from build123d import *

# Parameters (mm, degrees)
F0_R     = 10
F1_DEPTH = 20
F2_R     = 9
F3_DEPTH = 25


with BuildPart() as f1:
    # F0 (on Top) → F1 (new body)
    with BuildSketch(Plane.XY):
        with BuildLine():
            Line((0, -48.967767), (0, 0))
            Line((0, 0), (-150, 0))
            Line((-150, 0), (-150, -19.634434))
            ThreePointArc((-150, -19.634434), (-145.859777, -31.819157), (-135.153253, -38.959133))
            Line((-135.153253, -38.959133), (-25.153253, -68.292466))
            ThreePointArc((-25.153253, -68.292466), (-7.815277, -64.827544), (0, -48.967767))
        make_face()
        with Locations((-20, -48.967767)):
            Circle(F0_R, mode=Mode.SUBTRACT)
        with Locations((-130, -19.634434)):
            Circle(F0_R, mode=Mode.SUBTRACT)
    extrude(amount=F1_DEPTH)

    # F2 (on Front) → F3 (join)
    with BuildSketch(Plane.XZ):
        with BuildLine():
            Line((-84.449692, 0), (0, 0))
            Line((0, 0), (0, 35.662658))
            ThreePointArc((0, 35.662658), (-7.296527, 50.134551), (-23.270631, 52.873714))
            Line((-23.270631, 52.873714), (-75.468414, 36.888917))
            ThreePointArc((-75.468414, 36.888917), (-81.960416, 32.297455), (-84.449692, 24.745561))
            Line((-84.449692, 24.745561), (-84.449692, 0))
        make_face()
        with Locations((-16.808609, 38.975652)):
            Circle(F2_R, mode=Mode.SUBTRACT)
    extrude(amount=F3_DEPTH)


solid = f1.part
Work out the finished part from the listing and answer in its coordinate system (mm). A direction names the side the tool comes from. Coordinates: 2 decimals unless noted, no trailing zeros. Loops run counter-clockwise (first coordinate to the right, second up) from the corner with the lowest first, then second, coordinate; pieces in that order, holes last. Notation, with made-up numbers: M 86.25,7 L 90.25,7 A11 cw 90.25,15 Z; hole C -27.5,25 d1. An arc over 180 degrees is marked long. Answer in a Markdown table with one row per item. Add a question column.
1. Find section C-C, the plane y = -12. Write down the section's boundary in (x, z).
2. A tool of negligible diameter and unlimited length cuts with its end or side. For faces 1 (the cylindrical face through (-10.462, -45.964, 9.86)), 2 (the flat face through (-84.45, -12, 22)), 3 (the flat face through (-43, -25, 33)), from which of +Z, -Z, +X, -X, +Y, -Y can it reach the whole face along a straight path? Write none if from no direction.
3. Find section D-D, the plane x = -20. Write down the section's boundary in (y, z), then the cut area to 3 significant figures.
4. Find section B-B, the plane z = 32.5. Write down the section's boundary in (x, y).
5. The mould has two halves that part along X. Classify faces 4 (the cylindrical face through (-18.8, -12.3, 30.2)), 5 (the flat face through (-150, -10, 10)), 6 (the flat face through (0, -19, 14)): pulls with the +X half, pulls with the -X half, needs draft (parallel to the pull), parting line crosses it, or undercut.
6. Flat-ended cylindrical pins translate along their axes: P1, Ø10, axis at x = -54, z = 38, coming from the -Y side; P2, Ø2.5, axis at y = -7, z = 22.5, coming from the -X side; P3, Ø1, axis at x = -59, z = 16, coming from the -Y side; P4, Ø16, axis at x = -16.81, z = 38.98, coming from the +Y side. Find the tip coordinate at first contact, or state that the pin passes through.
7. Consider L1, parallel to Y at x = -20, z = 14; L2, parallel to Z at x = -113.5, y = -26.5; L3, parallel to X at y = -23.5, z = 11.5. Determine where each line is inside the solid, lowest interval first.
8. Find section A-A, the plane x = -127.5. Write down the section's boundary in (y, z), then the cut area to 3 significant figures.
Reported:
| question | item | result |
|---|---|---|
| 1 | outline | M -150,0 L -136.46,0 L -136.46,20 L -150,20 Z; M -123.54,0 L 0,0 L 0,35.66 A18 ccw -23.27,52.87 L -75.47,36.89 A12.7 ccw -84.45,24.75 L -84.45,20 L -123.54,20 Z; hole C -16.81,38.98 d18 |
| 2 | face 1 | +Z, -Z |
| 2 | face 2 | +Z, -X, +Y, -Y |
| 2 | face 3 | +Z, +X, -X, -Y |
| 3 | outline | M -68.97,0 L -58.97,0 L -58.97,20 L -68.97,20 Z; M -38.97,0 L 0,0 L 0,30.56 L -25,30.56 L -25,20 L -38.97,20 Z; M -25,47.39 L 0,47.39 L 0,53.55 L -25,53.55 Z |
| 3 | area | 1,400 mm^2 |
| 4 | outline | M -81.81,-25 L -23.06,-25 L -23.06,0 L -81.81,0 Z; M -10.56,-25 L 0,-25 L 0,0 L -10.56,0 Z |
| 5 | face 4 | undercut |
| 5 | face 5 | pulls with the -X half |
| 5 | face 6 | pulls with the +X half |
| 6 | P1 | stops at y = -25 |
| 6 | P2 | stops at x = -84.45 |
| 6 | P3 | stops at y = -59.4 |
| 6 | P4 | passes through |
| 7 | L1 | y = -68.97 to -58.97, -38.97 to 0 |
| 7 | L2 | z = 0 to 20 |
| 7 | L3 | x = -149.62 to -139.22, -120.78 to 0 |
| 8 | outline | M -41,0 L -29.32,0 L -29.32,20 L -41,20 Z; M -9.95,0 L 0,0 L 0,20 L -9.95,20 Z |
| 8 | area | 433 mm^2 |
